from build123d import *

# Parameters (mm, degrees)
F0_R     = 15
F0_R_2   = 5.9145568826
F1_DEPTH = 10
F0_R_3   = 5.8825208245
F2_R     = 6.5
F3_DEPTH = 215.6834155321


with BuildPart() as f1:
    # F0 (on Top) → F1 (new body, symmetric)
    with BuildSketch(Plane.XY):
        with Locations((-227.5, 0)):
            Circle(F0_R)
        with Locations((-227.5, 0)):
            Circle(F0_R_2, mode=Mode.SUBTRACT)
    extrude(amount=F1_DEPTH, both=True)



with BuildPart() as f1b:
    # F0 (on Top) → F1, piece 2 (new body, symmetric)
    with BuildSketch(Plane.XY):
        with Locations((227.5, 0)):
            Circle(F0_R)
        with Locations((227.5, 0)):
            Circle(F0_R_3, mode=Mode.SUBTRACT)
    extrude(amount=F1_DEPTH, both=True)


with BuildPart() as f1_1:
    add(f1.part)

    add(f1b.part)  # F3 merges F1b
    # F2 (on Right) → F3 (join, symmetric)
    with BuildSketch(Plane.YZ):
        Circle(F2_R)
    extrude(amount=F3_DEPTH, both=True)


solid = f1_1.part
The model under review builds one solid part; all positions refer to its coordinate system, in mm. Give positions to 0.01 mm unless a question says otherwise; leave off trailing zeros. Write each loop counter-clockwise with the first axis right and the second up, starting at its lowest first coordinate (ties: lowest second). Pieces come first, ordered by that corner, then holes.
1. Add section A-A, the plane x = -227.5. Write out the cut boundary in (y, z), plus the area to 3 significant figures.
2. Wall thickness on L1, parallel to Y at x = 227.5, z = -4.75; L2, parallel to X at y = 5, z = -5.25; L3, parallel to Z at x = 210.5, y = -1: over which ranges is each line inside the solid? List them lowest first.
3. Add section D-D, the plane x = 227.5. Write out the cut boundary in (y, z), plus the area to 3 significant figures.
4. Add section C-C, the plane z = 0. Write out the cut boundary in (x, y), plus the area to 3 significant figures.
5. Draft analysis for pull direction Y (two halves, no side actions). For faces 1 (the flat face through (234, 0, -10)), 2 (the cylindrical face through (2.996, -5.158, -3.955)), 3 (the cylindrical face through (221.623, 0.259, -0.14)), state which applies: +Y half, -Y half, draft (parallel to the pull), parting line (faces both ways), or undercut.
6. Add section B-B, the plane y = 0. Write out the cut boundary in (x, z), plus the area to 3 significant figures.
7. For P1, Ø2, axis at y = 7, z = -3.5, coming from the -X side; P2, Ø8, axis at x = 66.5, y = 1.5, coming from the -Z side; P3, Ø3, axis at x = -82.5, z = -4.5, coming from the +Y side, all flat-tipped, find the tip position at first contact; note any pin that passes through.
Worked answers:
1. outline: (-15, -10) - (-5.91, -10) - (-5.91, 10) - (-15, 10) - close; (5.91, -10) - (15, -10) - (15, 10) - (5.91, 10) - close
1. area: 363 mm2
2. L1: y = -15 to -5.88, 5.88 to 15
2. L2: x = -241.64 to -230.66, -224.34 to -213.36, 213.36 to 224.4, 230.6 to 241.64
2. L3: z = -6.42 to 6.42
3. outline: (-15, -10) - (-5.88, -10) - (-5.88, 10) - (-15, 10) - close; (5.88, -10) - (15, -10) - (15, 10) - (5.88, 10) - close
3. area: 365 mm2
4. outline: (-213.98, -6.5) - (213.98, -6.5) arc R15 ccw (long way) to (213.98, 6.5) - (-213.98, 6.5) arc R15 ccw (long way) to start; hole circle Ø11.83 at (-227.5, 0); hole circle Ø11.77 at (227.5, 0)
4. area: 6,730 mm2
5. face 1: draft
5. face 2: parting line
5. face 3: undercut
6. outline: (-242.5, -10) - (-233.41, -10) - (-233.41, 10) - (-242.5, 10) - close; (-221.59, -10) - (-212.5, -10) - (-212.5, -6.5) - (212.5, -6.5) - (212.5, -10) - (221.62, -10) - (221.62, 10) - (212.5, 10) - (212.5, 6.5) - (-212.5, 6.5) - (-212.5, 10) - (-221.59, 10) - close; (233.38, -10) - (242.5, -10) - (242.5, 10) - (233.38, 10) - close
6. area: 6,250 mm2
7. P1: stops at x = -241.25
7. P2: stops at z = -6.5
7. P3: stops at y = 5.77
